Source: CAD feature listing. Evaluate the final solid. Frame: model axes, mm. Face numbers are marked on the shaded views. A direction names the side the tool comes from. Round coordinates to 2 decimals unless told otherwise and drop trailing zeros. Write each loop counter-clockwise with the first axis right and the second up, starting at its lowest first coordinate (ties: lowest second). Pieces come first, ordered by that corner, then holes. Notation, with made-up numbers: (27, -36.75) -> (62, -36.75) arc R20 ccw to (62, -14.75) -> close; hole circle Ø9 at (-36, 0). An arc over 180 degrees is marked (long way). Put each result on its own line as item: value.
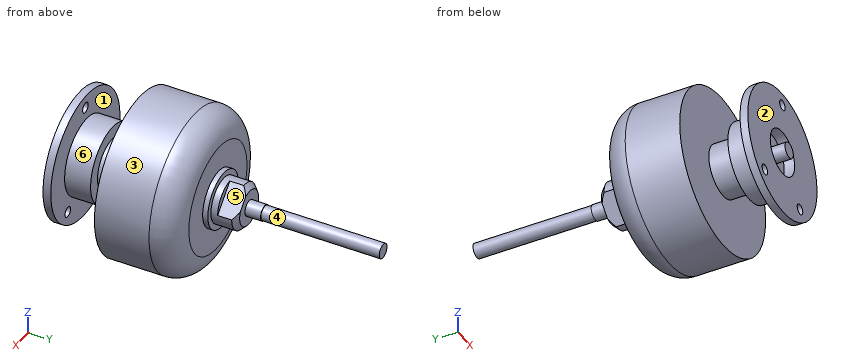
```python
from build123d import *

# Parameters (mm, degrees)
SKETCH1_R       = 12.5
EXTRUDE1_DEPTH  = 1.5
SKETCH2_R       = 7.5
EXTRUDE2_DEPTH  = 5
SKETCH3_R       = 5
EXTRUDE3_DEPTH  = 5
SKETCH4_R       = 15.5
EXTRUDE4_DEPTH  = 15.5
SKETCH5_R       = 5.5
EXTRUDE5_DEPTH  = 1
SKETCH6_R       = 4.4
EXTRUDE6_DEPTH  = 5
EXTRUDE7_START  = -3.7
EXTRUDE7_DEPTH  = 3.7
SKETCH8_R       = 1.5
EXTRUDE8_DEPTH  = 3
SKETCH9_R       = 1.4
EXTRUDE9_DEPTH  = 22.8
SKETCH10_R      = 4.4
EXTRUDE10_DEPTH = 2
EXTRUDE11_START = 3.3
SKETCH11_R      = 1.5
EXTRUDE11_DEPTH = 3.3
EXTRUDE12_REACH = 64.753
SKETCH12_R      = 1
FILLET1_R       = 5
CHAMFER1_SIZE   = 1


with BuildPart() as part:
    # Sketch1 → Extrude1 (new body)
    with BuildSketch(Plane(origin=(0, 0, 0), x_dir=(1, 0, 0), z_dir=(0, 1, 0))):
        with Locations(Location((0, 0, 0), (0, 0, 270))):
            Circle(SKETCH1_R)
    extrude(amount=EXTRUDE1_DEPTH)

    # Sketch2 → Extrude2 (add)
    with BuildSketch(Plane(origin=(0, 1.5, 0), x_dir=(1, 0, 0), z_dir=(0, 1, 0))):
        with Locations(Location((0, 0, 0), (0, 0, 270))):
            Circle(SKETCH2_R)
    extrude(amount=EXTRUDE2_DEPTH)

    # Sketch3 → Extrude3 (add)
    with BuildSketch(Plane(origin=(0, 6.5, 0), x_dir=(1, 0, 0), z_dir=(0, 1, 0))):
        with Locations(Location((0, 0, 0), (0, 0, 270))):
            Circle(SKETCH3_R)
    extrude(amount=EXTRUDE3_DEPTH)

    # Sketch4 → Extrude4 (add)
    with BuildSketch(Plane(origin=(0, 11.5, 0), x_dir=(1, 0, 0), z_dir=(0, 1, 0))):
        with Locations(Location((0, 0, 0), (0, 0, 270))):
            Circle(SKETCH4_R)
    extrude(amount=EXTRUDE4_DEPTH)

    # Sketch5 → Extrude5 (add)
    with BuildSketch(Plane(origin=(0, 27, 0), x_dir=(1, 0, 0), z_dir=(0, 1, 0))):
        with Locations(Location((0, 0, 0), (0, 0, 270))):
            Circle(SKETCH5_R)
    extrude(amount=EXTRUDE5_DEPTH)

    # Sketch6 → Extrude6 (add)
    with BuildSketch(Plane(origin=(0, 28, 0), x_dir=(1, 0, 0), z_dir=(0, 1, 0))):
        with Locations(Location((0, 0, 0), (0, 0, 270))):
            Circle(SKETCH6_R)
    extrude(amount=EXTRUDE6_DEPTH)

    # Sketch7 → Extrude7 (cut)
    with BuildSketch(Plane(origin=(0, 33, 0), x_dir=(1, 0, 0), z_dir=(0, 1, 0)).offset(EXTRUDE7_START)):
        with BuildLine():
            Line((0, 4.4), (-4.4, 0))
            ThreePointArc((-4.4, 0), (-3.111269837, 3.111269837), (0, 4.4))
        make_face()
        with BuildLine():
            Line((4.4, 0), (0, -4.4))
            ThreePointArc((0, -4.4), (3.111269837, -3.111269837), (4.4, 0))
        make_face()
    extrude(amount=EXTRUDE7_DEPTH, mode=Mode.SUBTRACT)

    # Sketch8 → Extrude8 (add)
    with BuildSketch(Plane(origin=(0, 33, 0), x_dir=(1, 0, 0), z_dir=(0, 1, 0))):
        with Locations(Location((0, 0, 0), (0, 0, 270))):
            Circle(SKETCH8_R)
    extrude(amount=EXTRUDE8_DEPTH)

    # Sketch9 → Extrude9 (add)
    with BuildSketch(Plane(origin=(0, 36, 0), x_dir=(1, 0, 0), z_dir=(0, 1, 0))):
        with Locations(Location((0, 0, 0), (0, 0, 270))):
            Circle(SKETCH9_R)
    extrude(amount=EXTRUDE9_DEPTH)

    # Sketch10 → Extrude10 (cut)
    with BuildSketch(Plane.XZ):
        with Locations(Location((0, 0, 0), (0, 0, 90))):
            Circle(SKETCH10_R)
    extrude(amount=-EXTRUDE10_DEPTH, mode=Mode.SUBTRACT)

    # Sketch11 → Extrude11 (add)
    with BuildSketch(Plane.XZ.offset(-2).offset(EXTRUDE11_START)):
        with Locations(Location((0, 0, 0), (0, 0, 90))):
            Circle(SKETCH11_R)
    extrude(amount=-EXTRUDE11_DEPTH)

    # Sketch12 → Extrude12 (cut, up to next)
    with BuildSketch(Plane.XZ, mode=Mode.PRIVATE) as extrude12_sk1:
        with Locations(Location((0, 10.102788136, 0), (0, 0, 270))):
            Circle(SKETCH12_R)
    extrude12_tool1 = extrude(extrude12_sk1.sketch, amount=-EXTRUDE12_REACH, mode=Mode.PRIVATE) & part.part
    # Sketch12 → Extrude12 (cut, up to next)
    with BuildSketch(Plane.XZ, mode=Mode.PRIVATE) as extrude12_sk2:
        with Locations(Location((-6.35, -7.857724106, 0), (0, 0, 270))):
            Circle(SKETCH12_R)
    extrude12_tool2 = extrude(extrude12_sk2.sketch, amount=-EXTRUDE12_REACH, mode=Mode.PRIVATE) & part.part
    # Sketch12 → Extrude12 (cut, up to next)
    with BuildSketch(Plane.XZ, mode=Mode.PRIVATE) as extrude12_sk3:
        with Locations(Location((6.35, -7.857724106, 0), (0, 0, 270))):
            Circle(SKETCH12_R)
    extrude12_tool3 = extrude(extrude12_sk3.sketch, amount=-EXTRUDE12_REACH, mode=Mode.PRIVATE) & part.part
    add(extrude12_tool1.solids().sort_by_distance((0, 0, 10.102788))[0], mode=Mode.SUBTRACT)
    add(extrude12_tool2.solids().sort_by_distance((-6.35, 0, -7.857724))[0], mode=Mode.SUBTRACT)
    add(extrude12_tool3.solids().sort_by_distance((6.35, 0, -7.857724))[0], mode=Mode.SUBTRACT)

    # Fillet1
    fillet1_edges = [part.edges().sort_by_distance(p)[0] for p in [
        (0, 27, -15.5),
    ]]
    fillet(fillet1_edges, radius=FILLET1_R)

    # Chamfer1
    chamfer1_edges = [part.edges().sort_by_distance(p)[0] for p in [
        (-3.111269837, 33, 3.111269837),
        (3.111269837, 33, -3.111269837),
    ]]
    chamfer(chamfer1_edges, length=CHAMFER1_SIZE)


solid = part.part
```
Q1. Cut plane A-A on x = 6.35. Give the number of separate pieces and of enclosed holes in the cut face, and give its area (3 significant figures).
Ans:
separate pieces: 3
enclosed holes: 0
area: 496 mm^2
Q2. Reachability of the marked faces 4, 5 and 6 from +Z, -Z, +X, -X, +Y, -Y: full face, straight path, thin tool, end or side. Return the list, or none.
Ans:
face 4: +Y
face 5: +Z, +X, +Y
face 6: none
Q3. Draft query along Y for the marked faces 1, 2 and 3. Return one class per face: +Y half, -Y half, draft (parallel to the pull), parting line (faces both ways), or undercut.
Ans:
face 1: undercut
face 2: -Y half
face 3: draft
Q4. Cut plane B-B on y = 49.5. Output: boundary loops of the cut face in (x, z), and give its area (3 significant figures).
Ans:
outline: circle Ø2.8 at (0, 0)
area: 6.16 mm^2
Q5. Material intervals for line 1 (X direction, y = 1.3, z = 0); line 2 (Y direction, x = 6.5, z = 5); line 3 (Y direction, x = -2.5, z = -11.5), sorted ascending. Write a range as [from, to].
Ans:
line 1: x = [-12.5, -4.4], [-1.5, 1.5], [4.4, 12.5]
line 2: y = [0, 1.5], [11.5, 27]
line 3: y = [0, 1.5], [11.5, 26.84]
Q6. Pin query (flat end, axial travel): pin 1 (1.5 mm diameter, centred on x = 7, y = 14, fed in from +Z); pin 2 (5 mm diameter, centred on y = 31.5, z = 1, fed in from -X); pin 3 (16.5 mm diameter, centred on x = 1.5, z = -3, fed in from +Y); pin 4 (3 mm diameter, centred on x = 6.35, z = -7.86, fed in from +Y). Return the tip coordinate at first contact, or that it passes through.
Ans:
pin 1: stops at z = 14.18
pin 2: stops at x = -4.4
pin 3: stops at y = 58.8
pin 4: stops at y = 27
